CAD build for the part. Positions are in the model's coordinates, mm. A direction names the side the tool comes from. Round coordinates to 2 decimals unless told otherwise and drop trailing zeros. Order: outer loops, then holes, each group sorted by start corner. A loop starts at its lowest first (then second) coordinate and runs counter-clockwise, first axis right, second up. Notation, with made-up numbers: (-7.5, 41.25) - (14.5, 41.25) arc R35 ccw to (14.5, 76.25) - close; hole circle Ø9 at (46, 0). An arc over 180 degrees is marked (long way). Write item = value, one per line.
from build123d import *

# Parameters (mm, degrees)
CUT_EXTRUDE3_DEPTH           = 60
CUT_EXTRUDE5_DEPTH           = 2
CUT_EXTRUDE5_DEPTH_BACK      = 30
SKETCH9_R                    = 38
SKETCH9_R_2                  = 23
SKETCH19_W                   = 12
SKETCH19_H                   = 36.5
CUT_REVOLVE2_ANGLE           = 65
CUT_REVOLVE2_OTHER_WAY_ANGLE = 65
SKETCH21_W                   = 3.25
SKETCH21_H                   = 4
BOSS_EXTRUDE3_DEPTH          = 1.35
CIRPATTERN1_COUNT            = 5
CUT_EXTRUDE9_START           = -5
CUT_EXTRUDE9_DEPTH           = 5
SKETCH23_R                   = 10.5
CUT_EXTRUDE10_DEPTH          = 10
SKETCH24_W                   = 15
SKETCH24_H                   = 8
BOSS_EXTRUDE4_DEPTH          = 8
SKETCH26_W                   = 10
SKETCH26_H                   = 6
CUT_EXTRUDE11_DEPTH          = 10
SKETCH27_W                   = 4
SKETCH27_H                   = 5
CUT_EXTRUDE12_DEPTH          = 5
CUT_EXTRUDE14_DEPTH          = 2
CUT_EXTRUDE14_DEPTH_BACK     = 30
SKETCH29_R                   = 1
CUT_EXTRUDE15_DEPTH          = 15
FILLET1_R                    = 6
FILLET2_R                    = 8
INTERSECT1_DEPTH             = 58.427876097
SKETCH31_W                   = 7
SKETCH31_H                   = 5
BOSS_EXTRUDE7_DEPTH          = 15
SKETCH32_R                   = 1.25
CUT_EXTRUDE16_DEPTH          = 7.5
FILLET3_R                    = 1


# Read off the part's stored shape, not the designer's step: Cut-Extrude9, Intersect1
with BuildPart() as part:
    # Sketch1 → Revolve1 (revolve)
    with BuildSketch(Plane.XY, mode=Mode.PRIVATE) as revolve1_sk:
        with BuildLine():
            Line((0, 63.427876097), (32, 63.427876097))
            ThreePointArc((32, 63.427876097), (37.656854249, 61.084730346), (40, 55.427876097))
            Line((40, 55.427876097), (40, 28.846818009))
            ThreePointArc((40, 28.846818009), (38.792081772, 24.082439968), (35.460140376, 20.469057744))
            Line((35.460140376, 20.469057744), (28.539859624, 15.958818353))
            ThreePointArc((28.539859624, 15.958818353), (25.207918228, 12.345436129), (24, 7.581058088))
            Line((24, 7.581058088), (24, 3.25))
            Line((24, 3.25), (24.35, 3))
            Line((24.35, 3), (24.35, 0))
            Line((24.35, 0), (22.5, 0))
            Line((22.5, 0), (22.5, 12.5))
            ThreePointArc((22.5, 12.5), (22.353553391, 12.853553391), (22, 13))
            Line((22, 13), (0, 13))
            Line((0, 13), (0, 63.427876097))
        make_face()
    revolve(revolve1_sk.sketch.rotate(Axis((0, 0, 0), (0, 1, 0)), 90), axis=Axis((0, 0, 0), (0, 1, 0)))

    # Sketch11 → Cut-Extrude3 (cut)
    with BuildSketch(Plane(origin=(0, 13, 0), x_dir=(-1, 0, 0), z_dir=(0, -1, 0))):
        with BuildLine():
            Line((-21, 0), (21, 0))
            ThreePointArc((21, 0), (0, 21), (-21, 0))
        make_face()
    extrude(amount=-CUT_EXTRUDE3_DEPTH, mode=Mode.SUBTRACT)

    # Sketch9 → Cut-Extrude5 (cut, two sides: drawn at the far end of the back side and taken through both)
    with BuildSketch(Plane(origin=(0, 55.427876097, 0), x_dir=(1, 0, 0), z_dir=(0, 1, 0)).offset(-CUT_EXTRUDE5_DEPTH_BACK)):
        with Locations(Location((0, 0, 0), (0, 0, 270))):
            Circle(SKETCH9_R)
        with Locations(Location((0, 0, 0), (0, 0, 270))):
            Circle(SKETCH9_R_2, mode=Mode.SUBTRACT)
    extrude(amount=CUT_EXTRUDE5_DEPTH + CUT_EXTRUDE5_DEPTH_BACK, mode=Mode.SUBTRACT)

    # Sketch19 → Cut-Revolve2 (revolve, cut)
    with BuildSketch(Plane(origin=(0, 0, 0), x_dir=(0, 0, -1), z_dir=(1, 0, 0))):
        with Locations((-41.064715832, 37.177876097)):
            Rectangle(SKETCH19_W, SKETCH19_H)
    revolve(axis=Axis((0, 0, 0), (0, 1, 0)), revolution_arc=CUT_REVOLVE2_ANGLE, mode=Mode.SUBTRACT)

    # Sketch19 → Cut-Revolve2 other way (revolve, cut)
    with BuildSketch(Plane(origin=(0, 0, 0), x_dir=(0, 0, -1), z_dir=(1, 0, 0))):
        with Locations((-41.064715832, 37.177876097)):
            Rectangle(SKETCH19_W, SKETCH19_H)
    revolve(axis=Axis((0, 0, 0), (0, -1, 0)), revolution_arc=CUT_REVOLVE2_OTHER_WAY_ANGLE, mode=Mode.SUBTRACT)

    # Sketch21 → Boss-Extrude3 (add)
    with BuildSketch(Plane(origin=(0, 0, 22.5), x_dir=(-1, 0, 0), z_dir=(0, 0, -1))):
        with Locations((0, 2)):
            Rectangle(SKETCH21_W, SKETCH21_H)
    boss_extrude3 = extrude(amount=BOSS_EXTRUDE3_DEPTH)

    # CirPattern1: Boss-Extrude3 ×5 about axis
    cirpattern1_axis = Axis((0, 0, 0), (0, 1, 0))
    for i in range(1, CIRPATTERN1_COUNT):
        add(boss_extrude3.rotate(cirpattern1_axis, i * 360 / CIRPATTERN1_COUNT))

    # Cut-Extrude9 outline → Cut-Extrude9 (cut)
    with BuildSketch(Plane(origin=(0, 63.427876097, 0), x_dir=(1, 0, 0), z_dir=(0, 1, 0)).offset(CUT_EXTRUDE9_START)):
        with BuildLine():
            ThreePointArc((40, 0), (0, 40), (-40, 0))
            Line((-40, 0), (-21, 0))
            ThreePointArc((-21, 0), (0, 21), (21, 0))
            Line((21, 0), (40, 0))
        make_face()
    extrude(amount=CUT_EXTRUDE9_DEPTH, mode=Mode.SUBTRACT)

    # Sketch23 → Cut-Extrude10 (cut)
    with BuildSketch(Plane(origin=(0, 0, -40), x_dir=(-1, 0, 0), z_dir=(0, 0, -1))):
        with Locations((0, 42.137876097)):
            Circle(SKETCH23_R)
    extrude(amount=-CUT_EXTRUDE10_DEPTH, mode=Mode.SUBTRACT)

    # Sketch24 → Boss-Extrude4 (add)
    with BuildSketch(Plane(origin=(0, 58.427876097, 0), x_dir=(1, 0, 0), z_dir=(0, 1, 0))):
        with Locations((0, 30)):
            Rectangle(SKETCH24_W, SKETCH24_H)
    extrude(amount=-BOSS_EXTRUDE4_DEPTH)

    # Sketch26 → Cut-Extrude11 (cut)
    with BuildSketch(Plane(origin=(0, 58.427876097, 0), x_dir=(1, 0, 0), z_dir=(0, 1, 0))):
        with Locations((0, 30)):
            Rectangle(SKETCH26_W, SKETCH26_H)
    extrude(amount=-CUT_EXTRUDE11_DEPTH, mode=Mode.SUBTRACT)

    # Sketch27 → Cut-Extrude12 (cut)
    with BuildSketch(Plane(origin=(7.5, 0, 0), x_dir=(0, 0, -1), z_dir=(1, 0, 0))):
        with Locations((30, 53.927876097)):
            Rectangle(SKETCH27_W, SKETCH27_H)
    extrude(amount=-CUT_EXTRUDE12_DEPTH, mode=Mode.SUBTRACT)

    # Sketch28 → Cut-Extrude14 (cut, two sides: drawn at the far end of the back side and taken through both)
    with BuildSketch(Plane(origin=(0, 55.427876097, 0), x_dir=(1, 0, 0), z_dir=(0, 1, 0)).offset(-CUT_EXTRUDE14_DEPTH_BACK)):
        with BuildLine():
            Line((-22.912878475, -2), (22.912878475, -2))
            ThreePointArc((22.912878475, -2), (0, -23), (-22.912878475, -2))
        make_face()
    extrude(amount=CUT_EXTRUDE14_DEPTH + CUT_EXTRUDE14_DEPTH_BACK, mode=Mode.SUBTRACT)

    # Sketch29 → Cut-Extrude15 (cut)
    with BuildSketch(Plane(origin=(0, 0, 0), x_dir=(-1, 0, 0), z_dir=(0, 0, -1))):
        with Locations((-30.416198487, 60.927876097)):
            Circle(SKETCH29_R)
        with Locations((30.416198487, 60.927876097)):
            Circle(SKETCH29_R)
        with Locations((0, 60.927876097)):
            Circle(SKETCH29_R)
    extrude(amount=-CUT_EXTRUDE15_DEPTH, mode=Mode.SUBTRACT)

    # Fillet1
    fillet1_edges = [part.edges().sort_by_distance(p)[0] for p in [
        (21, 35.713938048, 0),
        (-21, 35.713938048, 0),
    ]]
    fillet(fillet1_edges, radius=FILLET1_R)

    # Fillet2
    fillet2_edges = [part.edges().sort_by_distance(p)[0] for p in [
        (-22.912878475, 41.427876097, 2),
        (22.912878475, 41.427876097, 2),
    ]]
    fillet(fillet2_edges, radius=FILLET2_R)

    # Intersect1 outline → Intersect1 (cut)
    with BuildSketch(Plane(origin=(0, 0, 0), x_dir=(1, 0, 0), z_dir=(0, 1, 0))):
        with BuildLine():
            Line((-37.508702776, -13.895942431), (-42, -15.355253362))
            Line((-42, -15.355253362), (-42, -41))
            Line((-42, -41), (42, -41))
            Line((42, -41), (42, -15.355253362))
            Line((42, -15.355253362), (37.508702776, -13.895942431))
            ThreePointArc((37.508702776, -13.895942431), (0, 40), (-37.508702776, -13.895942431))
        make_face()
        with BuildLine():
            ThreePointArc((19.246817919, 8.4), (18.767687244, 2.713664655), (13.747727085, 0))
            Line((13.747727085, 0), (-13.747727085, 0))
            ThreePointArc((-13.747727085, 0), (-18.767687244, 2.713664655), (-19.246817919, 8.4))
            ThreePointArc((-19.246817919, 8.4), (0, 21), (19.246817919, 8.4))
        make_face(mode=Mode.SUBTRACT)
    extrude(amount=INTERSECT1_DEPTH, mode=Mode.SUBTRACT)

    # Sketch31 → Boss-Extrude7 (add)
    with BuildSketch(Plane(origin=(0, 58.427876097, 0), x_dir=(1, 0, 0), z_dir=(0, 1, 0))):
        with Locations((6.5, -29.5)):
            Rectangle(SKETCH31_W, SKETCH31_H)
    extrude(amount=-BOSS_EXTRUDE7_DEPTH)

    # Sketch32 → Cut-Extrude16 (cut)
    with BuildSketch(Plane(origin=(10, 0, 0), x_dir=(0, 0, -1), z_dir=(1, 0, 0))):
        with Locations((-29.5, 46.427876097)):
            Circle(SKETCH32_R)
    extrude(amount=-CUT_EXTRUDE16_DEPTH, mode=Mode.SUBTRACT)

    # Fillet3
    fillet3_edges = [part.edges().sort_by_distance(p)[0] for p in [
        (0, 58.427876097, 0),
    ]]
    fillet(fillet3_edges, radius=FILLET3_R)


solid = part.part
(1) Band-saw the part on A-A on x = 0. List the corners of the cut face in (y, z).
Solved:
outline = (58.43, 1) arc R1 ccw to (59.43, 0) - (59.93, 0) - (59.93, 15) - (61.93, 15) - (61.93, 0) - (63.43, 0) - (63.43, 32) arc R8 ccw to (58.43, 39.42) - close
(2) Pull direction Y, two halves, no side cores. Call faces 1 (the cylindrical face through (-30.2, 59.95, 7.4)), 2 (the flat face through (-30, 61, 15)), 3 (the flat face through (0, 63.428, 12)), 4 (the flat face through (1, 62, 0)): released by +Y, released by -Y, zero draft, split by the parting line, or undercut.
Solved:
face_1 = undercut
face_2 = undercut
face_3 = released by +Y
face_4 = zero draft
(3) Probe line 1 along Y through (x, z) = (0, 7.5); line 2 along Y through (x, z) = (-5, 18.5); line 3 along X through (y, z) = (60.25, 11). List the from-to ranges inside material, lowest first.
Solved:
line_1 = 58.43 to 59.93, 61.93 to 63.43
line_2 = 58.43 to 63.43
line_3 = -36.77 to -31.15, -29.68 to -0.74, 0.74 to 29.68, 31.15 to 36.77
(4) Drop flat-ended pins along their axis: pin 1 (4 mm diameter, centred on y = 48.5, z = 28.5, fed in from +X); pin 2 (12 mm diameter, centred on x = 17.5, z = 18.5, fed in from -Y); pin 3 (4 mm diameter, centred on x = 30.5, y = 59.5, fed in from +Z). Give the stop position or say it passes through.
Solved:
pin_1 = 10
pin_2 = 58.43
pin_3 = 26.9
(5) Band-saw the part on B-B on y = 50. List the corners of the cut face in (x, z).
Solved:
outline = (3, 27) - (10, 27) - (10, 32) - (3, 32) - close
(6) Tool access for faces 5 (the flat face through (3, 51, 30)), 6 (the flat face through (10, 51, 30)), 7 (the flat face through (6, 51, 27)), 8 (the flat face through (0, 61, 15)): list every direction of +Z, -Z, +X, -X, +Y, -Y with a clear straight run to the whole face (end or side of a thin tool).
Solved:
face_5 = +Z, -Z, -X, -Y
face_6 = +Z, -Z, +X, -Y
face_7 = -Z, +X, -X, -Y
face_8 = -Z
(7) Band-saw the part on C-C on z = 4. Count the separate pieces of the cut face and the enclosed holes in it, plus the area to 3 significant figures.
Solved:
separate_pieces = 1
enclosed_holes = 3
area = 362 mm²
